from build123d import *

# Parameters (mm, degrees)
FILLET2_R  = 2.4
SKETCH2_W  = 16
SKETCH2_H  = 2
SLOT_DEPTH = 1.9


with BuildPart() as part:
    # BodySke → Base-Revolve (revolve)
    with BuildSketch(Plane.XY, mode=Mode.PRIVATE) as base_revolve_sk:
        Polygon((4.8, 4), (4.8, 8), (0, 7.580054415), (0, 0), (14.8, 0), (14.8, 4), align=None)
    revolve(base_revolve_sk.sketch.rotate(Axis((-25.4, 0, 0), (1, 0, 0)), 90), axis=Axis((-25.4, 0, 0), (1, 0, 0)))  # turned: the seam where the file's is

    # Fillet2
    fillet2_edges = [part.edges().sort_by_distance(p)[0] for p in [
        (0, 0, -7.580054415),
    ]]
    fillet(fillet2_edges, radius=FILLET2_R)

    # Sketch2 → Slot (cut)
    with BuildSketch(Plane(origin=(0, 0, 0), x_dir=(0, 0, -1), z_dir=(1, 0, 0))):
        Rectangle(SKETCH2_W, SKETCH2_H)
    extrude(amount=SLOT_DEPTH, mode=Mode.SUBTRACT)


solid = part.part
Work out the finished part from the listing and answer in its coordinate system (mm). A direction names the side the tool comes from. Give positions to 0.01 mm unless a question says otherwise; leave off trailing zeros. Loops run counter-clockwise (first coordinate to the right, second up) from the corner with the lowest first, then second, coordinate; pieces in that order, holes last. Notation, with made-up numbers: (87.25, 6) - (136.25, 6) arc R19 ccw to (136.25, 30) - close; hole circle Ø2 at (-9.75, 57). An arc over 180 degrees is marked (long way). Answer in a Markdown table with one row per item. Add a question column.
Q1. A tool of negligible diameter and unlimited length cuts with its end or side. For faces 1 (the cylindrical face through (9.73, 3.905, -0.867)), 2 (the flat face through (0, -3, 0)), 3 (the flat face through (1, 1, 0)), from which of +Z, -Z, +X, -X, +Y, -Y can it reach the whole face along a straight path? Write none if from no direction.
Q2. The part is cut by section C-C (x = 7). Determine the outline of the cut face in (y, z).
Q3. The part is cut by section D-D (x = 3). Determine the outline of the cut face in (y, z).
Q4. Determine the mould class of faces 4 (the conical face through (2.897, -2.353, 7.472)), 5 (the flat face through (0, 3, 0)), 6 (the flat face through (1, -1, 0)), 7 (the flat face through (1.9, 0, 0)) for opening direction Y: released by +Y, released by -Y, zero draft, split by the parting line, or undercut.
Q5. The part is cut by section B-B (y = 0). Determine the outline of the cut face in (x, z), and give its area (3 significant figures).
Q6. Each of these flat-tipped pins is pushed along its axis until it touches: P1, Ø0.6, axis at y = 0, z = 0, coming from the -X side; P2, Ø1.5, axis at x = 1, z = -2, coming from the +Y side; P3, Ø1.5, axis at x = 9.5, y = -0.5, coming from the +Z side. Where does it stop, or does it pass through?
Q7. The part is cut by section A-A (z = 0). Determine the outline of the cut face in (x, y).
Q8. Consider line 1 along X through (y, z) = (4, -2); line 2 along X through (y, z) = (0, -1); line 3 along Y through (x, z) = (2, -0.25). Determine where each line is inside the solid, lowest interval first.
Solution:
| question | item | result |
|---|---|---|
| 1 | face 1 | +X |
| 1 | face 2 | +Z, -Z, -X, +Y, -Y |
| 1 | face 3 | +Z, -Z, -X |
| 2 | outline | circle Ø8 at (0, 0) |
| 3 | outline | circle Ø15.69 at (0, 0) |
| 4 | face 4 | split by the parting line |
| 4 | face 5 | zero draft |
| 4 | face 6 | undercut |
| 4 | face 7 | undercut |
| 5 | outline | (1.9, -7.73) arc R2.4 ccw to (2.19, -7.77) - (4.8, -8) - (4.8, -4) - (14.8, -4) - (14.8, 4) - (4.8, 4) - (4.8, 8) - (2.19, 7.77) arc R2.4 ccw to (1.9, 7.73) - close |
| 5 | area | 126 mm² |
| 6 | P1 | stops at x = 1.9 |
| 6 | P2 | stops at y = 7.49 |
| 6 | P3 | stops at z = 4 |
| 7 | outline | (0, -5.38) arc R2.4 ccw to (2.19, -7.77) - (4.8, -8) - (4.8, -4) - (14.8, -4) - (14.8, 4) - (4.8, 4) - (4.8, 8) - (2.19, 7.77) arc R2.4 ccw to (0, 5.38) - (0, 1) - (1.9, 1) - (1.9, -1) - (0, -1) - close |
| 8 | line 1 | x = 0 to 4.8 |
| 8 | line 2 | x = 1.9 to 14.8 |
| 8 | line 3 | y = -7.74 to 7.74 |
